Check sheet for the modelled part. Datum: model origin and axes. Units: mm. Round coordinates to 2 decimals unless told otherwise and drop trailing zeros. Write each loop counter-clockwise with the first axis right and the second up, starting at its lowest first coordinate (ties: lowest second). Pieces come first, ordered by that corner, then holes. Notation, with made-up numbers: M 18,7.25 L 24,7.25 A20 cw 24,18.25 Z; hole C 85,-19.5 d2. An arc over 180 degrees is marked long. Answer in a Markdown table with one row per item.
```python
from build123d import *

# Parameters (mm, degrees)
F0_R     = 1.5
F1_DEPTH = 2


with BuildPart() as f1:
    # F0 (on Top) → F1 (new body)
    with BuildSketch(Plane.XY):
        with BuildLine():
            Line((-12, -15), (12, -15))
            ThreePointArc((12, -15), (14.12132, -14.12132), (15, -12))
            Line((15, -12), (15, 12))
            ThreePointArc((15, 12), (14.12132, 14.12132), (12, 15))
            Line((12, 15), (-12, 15))
            ThreePointArc((-12, 15), (-14.12132, 14.12132), (-15, 12))
            Line((-15, 12), (-15, -12))
            ThreePointArc((-15, -12), (-14.12132, -14.12132), (-12, -15))
        make_face()
        with Locations((-10, -10)):
            Circle(F0_R, mode=Mode.SUBTRACT)
        with Locations((-5, -10)):
            Circle(F0_R, mode=Mode.SUBTRACT)
        with Locations((0, -10)):
            Circle(F0_R, mode=Mode.SUBTRACT)
        with Locations((-10, -5)):
            Circle(F0_R, mode=Mode.SUBTRACT)
        with Locations((-5, -5)):
            Circle(F0_R, mode=Mode.SUBTRACT)
        with Locations((0, -5)):
            Circle(F0_R, mode=Mode.SUBTRACT)
        with Locations((5, -10)):
            Circle(F0_R, mode=Mode.SUBTRACT)
        with Locations((10, -10)):
            Circle(F0_R, mode=Mode.SUBTRACT)
        with Locations((5, -5)):
            Circle(F0_R, mode=Mode.SUBTRACT)
        with Locations((10, -5)):
            Circle(F0_R, mode=Mode.SUBTRACT)
        with Locations((-10, 0)):
            Circle(F0_R, mode=Mode.SUBTRACT)
        with Locations((-10, 5)):
            Circle(F0_R, mode=Mode.SUBTRACT)
        with Locations((-5, 0)):
            Circle(F0_R, mode=Mode.SUBTRACT)
        Circle(F0_R, mode=Mode.SUBTRACT)
        with Locations((-5, 5)):
            Circle(F0_R, mode=Mode.SUBTRACT)
        with Locations((0, 5)):
            Circle(F0_R, mode=Mode.SUBTRACT)
        with Locations((-10, 10)):
            Circle(F0_R, mode=Mode.SUBTRACT)
        with Locations((-5, 10)):
            Circle(F0_R, mode=Mode.SUBTRACT)
        with Locations((0, 10)):
            Circle(F0_R, mode=Mode.SUBTRACT)
        with Locations((5, 0)):
            Circle(F0_R, mode=Mode.SUBTRACT)
        with Locations((5, 5)):
            Circle(F0_R, mode=Mode.SUBTRACT)
        with Locations((10, 0)):
            Circle(F0_R, mode=Mode.SUBTRACT)
        with Locations((10, 5)):
            Circle(F0_R, mode=Mode.SUBTRACT)
        with Locations((5, 10)):
            Circle(F0_R, mode=Mode.SUBTRACT)
        with Locations((10, 10)):
            Circle(F0_R, mode=Mode.SUBTRACT)
    extrude(amount=F1_DEPTH)


solid = f1.part
```
1. Go/stop test with flat-tipped pins: pin 1 (2.5 mm diameter, centred on x = 5, y = 0, fed in from -Z); pin 2 (4 mm diameter, centred on x = 10, y = 10, fed in from +Z). Record where each tip stops, or that it passes through.
Found:
| item | result |
|---|---|
| pin 1 | passes through |
| pin 2 | stops at z = 2 |
2. Draft check along Y on faces 1 (the face through (-0.195, -3.513, 0.986)), 2 (the face through (-14.14, -14.1, 0.99)), 3 (the face through (3, 0, 2)). Enter one of: +Y half, -Y half, draft (parallel to the pull), parting line (faces both ways), or undercut.
Found:
| item | result |
|---|---|
| face 1 | undercut |
| face 2 | -Y half |
| face 3 | draft |
3. Scan lines: L1, parallel to Y at x = 5, z = 1.35; L2, parallel to Y at x = -11, z = 1.7; L3, parallel to X at y = -4.75, z = 1.2. Record each from-to range of solid material in increasing order.
Found:
| item | result |
|---|---|
| L1 | y = -15 to -11.5, -8.5 to -6.5, -3.5 to -1.5, 1.5 to 3.5, 6.5 to 8.5, 11.5 to 15 |
| L2 | y = -15 to -11.12, -8.88 to -6.12, -3.88 to -1.12, 1.12 to 3.88, 6.12 to 8.88, 11.12 to 15 |
| L3 | x = -15 to -11.48, -8.52 to -6.48, -3.52 to -1.48, 1.48 to 3.52, 6.48 to 8.52, 11.48 to 15 |
4. Section check A-A, the plane y = -5. Record the cut outline in (x, z), and give its area (3 significant figures).
Found:
| item | result |
|---|---|
| outline | M -15,0 L -11.5,0 L -11.5,2 L -15,2 Z; M -8.5,0 L -6.5,0 L -6.5,2 L -8.5,2 Z; M -3.5,0 L -1.5,0 L -1.5,2 L -3.5,2 Z; M 1.5,0 L 3.5,0 L 3.5,2 L 1.5,2 Z; M 6.5,0 L 8.5,0 L 8.5,2 L 6.5,2 Z; M 11.5,0 L 15,0 L 15,2 L 11.5,2 Z |
| area | 30.0 mm2 |
5. Section check C-C, the plane z = 1.3. Count the separate pieces of the cut face and the enclosed holes in it, and give its area (3 significant figures).
Found:
| item | result |
|---|---|
| separate pieces | 1 |
| enclosed holes | 25 |
| area | 716 mm2 |
